Drawing for the job (mm, zero at the part's lowest x, y, z). Round coordinates to 2 decimals unless told otherwise and drop trailing zeros. Write each loop counter-clockwise with the first axis right and the second up, starting at its lowest first coordinate (ties: lowest second). Pieces come first, ordered by that corner, then holes. Notation, with made-up numbers: (70.5, 38) -> (112.5, 38) arc R27 cw to (112.5, 61) -> close; hole circle Ø6 at (22, -18). An arc over 180 degrees is marked (long way). One line per question, with ' | ' between items.
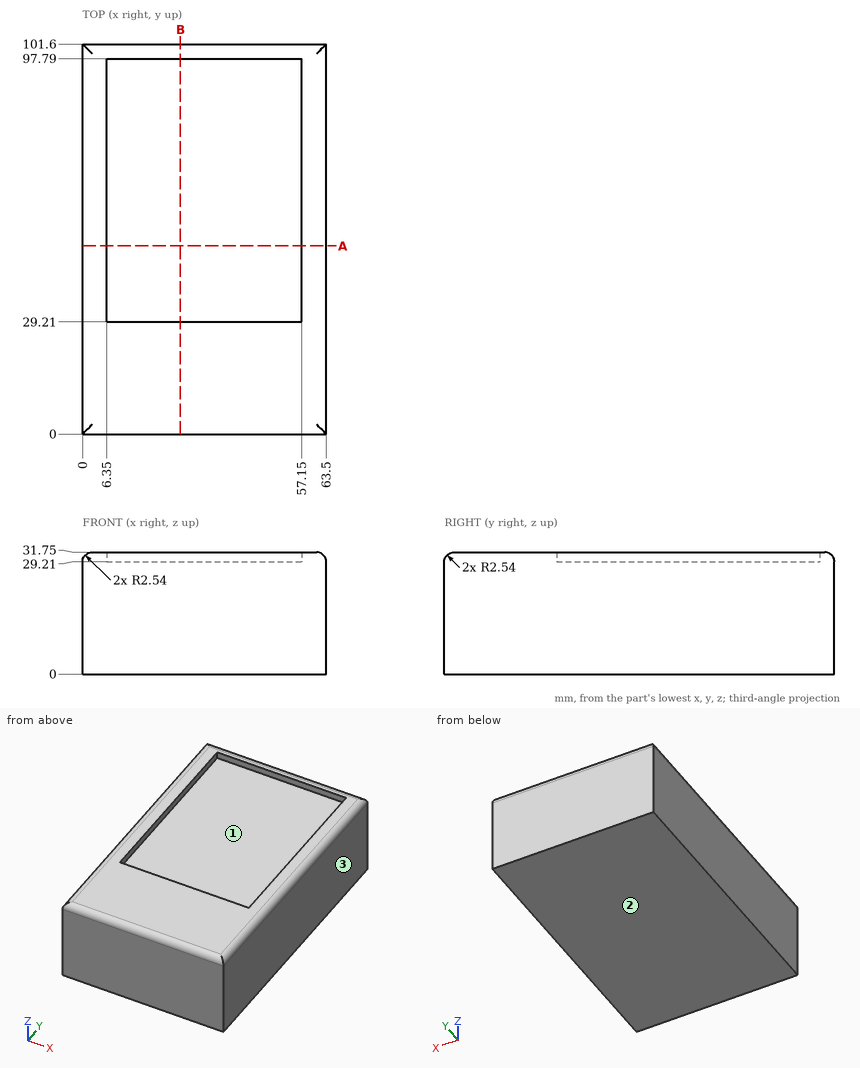
(1) Slice it at B-B (x = 25.5). Write the cut outline in (y, z), then the cut area to 3 significant figures.
Calculated:
outline: (0, 0) -> (101.6, 0) -> (101.6, 29.21) arc R2.54 ccw to (99.06, 31.75) -> (97.79, 31.75) -> (97.79, 29.21) -> (29.21, 29.21) -> (29.21, 31.75) -> (2.54, 31.75) arc R2.54 ccw to (0, 29.21) -> close | area: 3,050 mm2
(2) Wall check: line 1 (Y direction, x = 48, z = 30); line 2 (Z direction, x = 25.5, y = 56.5). Give the ranges that are in metal, low to high. Write a range as from..to.
Calculated:
line 1: 0.13..29.21, 97.79..101.47 | line 2: 0..29.21
(3) Drop flat-ended pins along their axis: pin 1 (1.3 mm diameter, centred on y = 68, z = 30.5, fed in from -X); pin 2 (2 mm diameter, centred on x = 29.5, z = 30.5, fed in from +Y); pin 3 (0.8 mm diameter, centred on x = 40.5, z = 30.5, fed in from -Y). Give the stop position or say it passes through.
Calculated:
pin 1: x = 0.08 | pin 2: y = 101.58 | pin 3: y = 0.16
(4) Mould opens along X. For the marked faces 1, 2 and 3 say: pulls with the +X half, pulls with the -X half, needs draft (parallel to the pull), parting line crosses it, or undercut.
Calculated:
face 1: undercut | face 2: needs draft | face 3: pulls with the +X half
(5) Slice it at A-A (y = 49). Write the cut outline in (x, z).
Calculated:
outline: (0, 0) -> (63.5, 0) -> (63.5, 29.21) arc R2.54 ccw to (60.96, 31.75) -> (57.15, 31.75) -> (57.15, 29.21) -> (6.35, 29.21) -> (6.35, 31.75) -> (2.54, 31.75) arc R2.54 ccw to (0, 29.21) -> close
